from build123d import *

# Parameters (mm, degrees)
SKETCH_3_R          = 6.75
CUT_EXTRUDE_1_DEPTH = 0.2
CUT_EXTRUDE_2_DEPTH = 0.2
SKETCH_5_R          = 7.3
CUT_EXTRUDE_3_DEPTH = 0.2
EXTRUDE_1_DEPTH     = 1.2
SKETCH_7_R          = 0.4
EXTRUDE_2_DEPTH     = 5.2


with BuildPart() as part:
    # Эскиз2 → Повернуть1 (revolve)
    with BuildSketch(Plane.XY):
        with BuildLine():
            Line((0, 0), (8.5, 0))
            ThreePointArc((8.5, 0), (9.207106781, 0.292893219), (9.5, 1))
            ThreePointArc((9.5, 1), (9.4701425, 1.242535625), (9.382352941, 1.470588235))
            ThreePointArc((9.382352941, 1.470588235), (9, 3), (9.382352941, 4.529411765))
            ThreePointArc((9.382352941, 4.529411765), (9.4701425, 4.757464375), (9.5, 5))
            Line((9.5, 5), (9.5, 40.5))
            ThreePointArc((9.5, 40.5), (9.207106781, 41.207106781), (8.5, 41.5))
            Line((8.5, 41.5), (0, 41.5))
            Line((0, 41.5), (0, 0))
        make_face()
    revolve(axis=Axis((0, 0, 0), (0, 1, 0)))

    # Эскиз3 → Вырез-Вытянуть1 (cut)
    with BuildSketch(Plane(origin=(0, 41.5, 0), x_dir=(1, 0, 0), z_dir=(0, 1, 0))):
        with Locations(Location((0, 0, 0), (0, 0, 180))):
            Circle(SKETCH_3_R)
    extrude(amount=-CUT_EXTRUDE_1_DEPTH, mode=Mode.SUBTRACT)

    # Эскиз4 → Вырез-Вытянуть2 (cut)
    with BuildSketch(Plane(origin=(0, 41.3, 0), x_dir=(1, 0, 0), z_dir=(0, 1, 0))):
        with BuildLine():
            Line((-0.25, -0.25), (-0.25, -5.76))
            ThreePointArc((-0.25, -5.76), (-0.179705627, -5.929705627), (-0.01, -6))
            Line((-0.01, -6), (0.01, -6))
            ThreePointArc((0.01, -6), (0.179705627, -5.929705627), (0.25, -5.76))
            Line((0.25, -5.76), (0.25, -0.25))
            Line((0.25, -0.25), (5.76, -0.25))
            ThreePointArc((5.76, -0.25), (5.929705627, -0.179705627), (6, -0.01))
            Line((6, -0.01), (6, 0.01))
            ThreePointArc((6, 0.01), (5.929705627, 0.179705627), (5.76, 0.25))
            Line((5.76, 0.25), (0.25, 0.25))
            Line((0.25, 0.25), (0.25, 5.76))
            ThreePointArc((0.25, 5.76), (0.179705627, 5.929705627), (0.01, 6))
            Line((0.01, 6), (-0.01, 6))
            ThreePointArc((-0.01, 6), (-0.179705627, 5.929705627), (-0.25, 5.76))
            Line((-0.25, 5.76), (-0.25, 0.25))
            Line((-0.25, 0.25), (-5.76, 0.25))
            ThreePointArc((-5.76, 0.25), (-5.929705627, 0.179705627), (-6, 0.01))
            Line((-6, 0.01), (-6, -0.01))
            ThreePointArc((-6, -0.01), (-5.929705627, -0.179705627), (-5.76, -0.25))
            Line((-5.76, -0.25), (-0.25, -0.25))
        make_face()
    extrude(amount=-CUT_EXTRUDE_2_DEPTH, mode=Mode.SUBTRACT)

    # Эскиз5 → Вырез-Вытянуть3 (cut)
    with BuildSketch(Plane.XZ):
        Circle(SKETCH_5_R)
    extrude(amount=-CUT_EXTRUDE_3_DEPTH, mode=Mode.SUBTRACT)

    # Эскиз6 → Бобышка-Вытянуть1 (add)
    with BuildSketch(Plane.XZ.offset(-0.2)):
        with BuildLine():
            Line((-5.337602458, 2), (5.337602458, 2))
            ThreePointArc((5.337602458, 2), (0, 5.7), (-5.337602458, 2))
        make_face()
        with BuildLine():
            Line((-5.337602458, -2), (5.337602458, -2))
            ThreePointArc((5.337602458, -2), (0, -5.7), (-5.337602458, -2))
        make_face()
    extrude(amount=EXTRUDE_1_DEPTH)

    # Эскиз7 → Бобышка-Вытянуть2 (add)
    with BuildSketch(Plane.XZ.offset(-0.2)):
        with Locations((-3.75, 0)):
            Circle(SKETCH_7_R)
        with Locations((3.75, 0)):
            Circle(SKETCH_7_R)
    extrude(amount=EXTRUDE_2_DEPTH)


solid = part.part
The listing builds one solid part. Answer for the finished solid, in the listing's coordinates (mm). A direction names the side the tool comes from. Round coordinates to 2 decimals unless told otherwise and drop trailing zeros. Order: outer loops, then holes, each group sorted by start corner. A loop starts at its lowest first (then second) coordinate and runs counter-clockwise, first axis right, second up. Notation, with made-up numbers: (40.5, 28.25) - (61.5, 28.25) arc R27 ccw to (61.5, 65.25) - close; hole circle Ø10 at (-39, 59). An arc over 180 degrees is marked (long way). Write item = value, one per line. Start each with the question number.
1) Given pin 1 (6 mm diameter, centred on x = 3.5, y = 11.5, fed in from +Z); pin 2 (6 mm diameter, centred on x = -2.5, z = -1, fed in from +Y); pin 3 (1.1 mm diameter, centred on x = 0, z = -4, fed in from -Y), each flat-ended and moving along its own axis, determine where each tip first touches the part or whether it passes through.
2) Section A-A, the plane y = 30 is taken. Write down the section's boundary in (x, z), plus the area to 3 significant figures.
3) For a pull along Z with two mould halves and no side action, classify faces 5 (the flat face through (3, 0, -7)), 6 (the flat face through (-1, 41.3, -1)), 7 (the cylindrical face through (4.38, 23, 8.43)) as released by +Z, released by -Z, zero draft, split by the parting line, or undercut.
4) For faces 1 (the flat face through (0, -1, -3)), 2 (the flat face through (0, 0, 2)), 3 (the flat face through (0, -1, 3)), 4 (the flat face through (1, 41.5, -7)), determine the directions among +Z, -Z, +X, -X, +Y, -Y from which every point of the face is accessible in a straight line to the end or side of a thin tool.
5) Straight lines are drawn through the part: L1, parallel to Z at x = 0, y = 0.1; L2, parallel to Y at x = -2.75, z = -5.5; L3, parallel to Y at x = -1, z = -8.5. For each, find the intervals that lie inside material, in ascending order.
Results list:
q1.pin_1 = 9.49
q1.pin_2 = 41.3
q1.pin_3 = -1
q2.outline = circle Ø19 at (0, 0)
q2.area = 284 mm^2
q3.face_5 = zero draft
q3.face_6 = undercut
q3.face_7 = split by the parting line
q4.face_1 = -Z, +X, -X, -Y
q4.face_2 = -Y
q4.face_3 = +Z, +X, -X, -Y
q4.face_4 = +Z, -Z, +X, -X, +Y
q5.L1 = -8.94 to -7.3, -5.7 to -2, 2 to 5.7, 7.3 to 8.94
q5.L2 = 0.2 to 41.3
q5.L3 = 0 to 41.5
